The model under review builds one solid part; all positions refer to its coordinate system, in mm. Face numbers are marked on the shaded views. A direction names the side the tool comes from. Round coordinates to 2 decimals unless told otherwise and drop trailing zeros. Write each loop counter-clockwise with the first axis right and the second up, starting at its lowest first coordinate (ties: lowest second). Pieces come first, ordered by that corner, then holes.
Item 1: Add section D-D (y = 50.5). Give the boundary of the cut face in (x, z) (3 decimals), plus the area to 3 significant figures.
Item 2: To check wall thickness, follow L1, parallel to Y at x = -101.6, z = -26.5; L2, parallel to Z at x = 16.5, y = -34 (3 decimals). State the ranges of each line that lie inside material, in increasing order.
Item 3: Add section A-A (x = 0). State how many separate pieces and enclosed holes the cut face has, plus the area to 3 significant figures.
Item 4: Clearance check with flat-ended pins moving along their axes: pin 1 Ø5 at (y, z) = (-44, -1) entering from -X; pin 2 Ø10 at (x, y) = (-93.5, -20.5) entering from +Z; pin 3 Ø12.5 at (x, y) = (0, 31.75) entering from -Z. State where each tip first meets the part, or that it passes through.
Item 5: Add section C-C (x = 51). Give the boundary of the cut face in (y, z).
Item 6: Draft analysis for pull direction X (two halves, no side actions). For the marked faces 1, 2 and 3, state which applies: +X half, -X half, draft (parallel to the pull), parting line (faces both ways), or undercut.
Item 7: Machinability: for the marked faces 4, 5 and 6, which of the approach directions +Z, -Z, +X, -X, +Y, -Y give a long, thin tool a straight path to every point of the face, cutting with its end or side? Answer none if there is none.
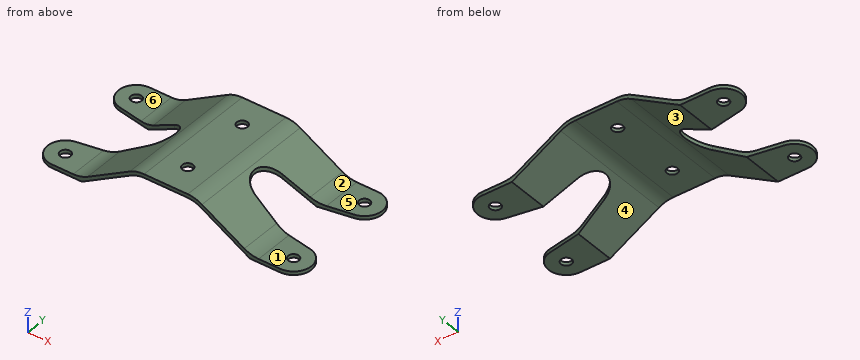
```python
from build123d import *

# Parameters (mm, degrees)
F1_DEPTH      = 63.5
F1_DEPTH_BACK = 74.676
F3_START      = -145.542
F2_R          = 4.7625
F3_DEPTH      = 250.19
F4_R          = 25.4


with BuildPart() as f1:
    # F0 (on Front) → F1 (new body, two sides)
    with BuildSketch(Plane.XZ) as f1_sk:
        Polygon((-25.4, 0), (0, 0), (25.4, 0), (74.8933518263, -28.575), (127, -28.575), (127, -25.4), (75.7440905122, -25.4), (26.250738686, 3.175), (0, 3.175), (-26.250738686, 3.175), (-75.7440905122, -25.4), (-127, -25.4), (-127, -28.575), (-74.8933518263, -28.575), align=None)
    extrude(amount=F1_DEPTH)
    extrude(f1_sk.sketch, amount=-F1_DEPTH_BACK)

    # F2 (on Top) → F3 (intersect)
    with BuildSketch(Plane.XY.offset(F3_START)):
        with BuildLine():
            ThreePointArc((-104.0748523501, -25.594096619), (-117.4264014573, -42.5162259718), (-101.6, -57.15))
            Line((-101.6, -57.15), (0, -57.15))
            Line((0, -57.15), (101.6, -57.15))
            ThreePointArc((101.6, -57.15), (117.4264014573, -42.5162259718), (104.0748523501, -25.594096619))
            Line((104.0748523501, -25.594096619), (48.2385059171, -15.6280150973))
            ThreePointArc((48.2385059171, -15.6280150973), (35.1529089212, 0), (48.2385059171, 15.6280150973))
            Line((48.2385059171, 15.6280150973), (104.0748523501, 25.594096619))
            ThreePointArc((104.0748523501, 25.594096619), (117.4264014573, 42.5162259718), (101.6, 57.15))
            Line((101.6, 57.15), (0, 57.15))
            Line((0, 57.15), (-101.6, 57.15))
            ThreePointArc((-101.6, 57.15), (-117.4264014573, 42.5162259718), (-104.0748523501, 25.594096619))
            Line((-104.0748523501, 25.594096619), (-48.2385059171, 15.6280150973))
            ThreePointArc((-48.2385059171, 15.6280150973), (-35.1529089212, 0), (-48.2385059171, -15.6280150973))
            Line((-48.2385059171, -15.6280150973), (-104.0748523501, -25.594096619))
        make_face()
        with Locations((-101.6, -41.275)):
            Circle(F2_R, mode=Mode.SUBTRACT)
        with Locations((0, -31.75)):
            Circle(F2_R, mode=Mode.SUBTRACT)
        with Locations((101.6, -41.275)):
            Circle(F2_R, mode=Mode.SUBTRACT)
        with Locations((-101.6, 41.275)):
            Circle(F2_R, mode=Mode.SUBTRACT)
        with Locations((0, 31.75)):
            Circle(F2_R, mode=Mode.SUBTRACT)
        with Locations((101.6, 41.275)):
            Circle(F2_R, mode=Mode.SUBTRACT)
    extrude(amount=F3_DEPTH, mode=Mode.INTERSECT)

    # F4
    f4_edges = [f1.edges().sort_by_distance(p)[0] for p in [
        (-75.744091, -38.843707, -25.4),
        (-75.744091, 38.843707, -25.4),
        (-26.250739, 0, 3.175),
        (26.250739, 0, 3.175),
        (75.744091, -38.843707, -25.4),
        (75.744091, 38.843707, -25.4),
        (-25.4, 0, 0),
        (25.4, 0, 0),
    ]]
    fillet(f4_edges, radius=F4_R)


solid = f1.part
```
Numbers:
1. outline: (-114.52, -28.575) - (-74.893, -28.575) - (-31.294, -3.403) arc R25.4 cw to (-18.594, 0) - (18.594, 0) arc R25.4 cw to (31.294, -3.403) - (74.893, -28.575) - (114.52, -28.575) - (114.52, -25.4) - (82.55, -25.4) arc R25.4 cw to (69.85, -21.997) - (32.145, -0.228) arc R25.4 ccw to (19.445, 3.175) - (-19.445, 3.175) arc R25.4 ccw to (-32.145, -0.228) - (-69.85, -21.997) arc R25.4 cw to (-82.55, -25.4) - (-114.52, -25.4) - close
1. area: 784 mm2
2. L1: y = -57.15 to -46.04, -36.51 to -25.15, 25.15 to 36.51, 46.04 to 57.15
2. L2: z = 0 to 3.175
3. separate pieces: 3
3. enclosed holes: 0
3. area: 302 mm2
4. pin 1: stops at x = -37.81
4. pin 2: stops at z = -25.4
4. pin 3: stops at z = 0
5. outline: (-57.15, -14.78) - (-16.12, -14.78) - (-16.12, -11.11) - (-57.15, -11.11) - close; (16.12, -14.78) - (57.15, -14.78) - (57.15, -11.11) - (16.12, -11.11) - close
6. face 1: draft
6. face 2: +X half
6. face 3: undercut
7. face 4: -Z, +Y, -Y
7. face 5: +Z, +X, +Y, -Y
7. face 6: +Z, -X, +Y, -Y
